Geometry check sheet. Reference: the model listing, model coordinates, mm. Face numbers are marked on the shaded views. A direction names the side the tool comes from. Coordinates: 2 decimals unless noted, no trailing zeros. Order: outer loops, then holes, each group sorted by start corner. A loop starts at its lowest first (then second) coordinate and runs counter-clockwise, first axis right, second up. Notation, with made-up numbers: M 21,-17.5 L 51,-17.5 A6 ccw 51,-12.5 Z; hole C -17.5,46.5 d5. An arc over 180 degrees is marked long. Use CSV: the item, a comma, the result in double quotes. Start each with the question number.
```python
from build123d import *

# Parameters (mm, degrees)
F3_DEPTH = 3.175
F5_DEPTH = 1.27
F6_SIZE2 = 1.27
F6_SIZE  = 0.7332348419


with BuildPart() as f1:
    # F0 (on Top) → F1 (revolve)
    with BuildSketch(Plane.XY):
        Polygon((0, 3.429), (0, 10.2616), (-6.35, 10.2616), (-6.35, 2.38125), (-3.175, 2.38125), (-3.175, 4.191), (-1.905, 4.191), (-1.905, 3.429), align=None)
    revolve(axis=Axis((-3.175, 0, 0), (-1, 0, 0)))

    # F2 (on face) → F3 (cut, through all)
    with BuildSketch(Plane.YZ):
        with BuildLine():
            ThreePointArc((3.429, 0), (2.4246691527, -2.4246691527), (0, -3.429))
            Line((0, -3.429), (9.6717316733, -3.429))
            ThreePointArc((9.6717316733, -3.429), (10.1130578041, -1.7396828477), (10.2616, 0))
            ThreePointArc((10.2616, 0), (10.1130578041, 1.7396828477), (9.6717316733, 3.429))
            Line((9.6717316733, 3.429), (0, 3.429))
            ThreePointArc((0, 3.429), (2.4246691527, 2.4246691527), (3.429, 0))
        make_face()
    extrude(amount=-F3_DEPTH, mode=Mode.SUBTRACT)

    # F4 (on face) → F5 (cut)
    with BuildSketch(Plane.YZ.offset(-3.175)):
        with BuildLine():
            ThreePointArc((0, 4.191), (-4.191, 0), (0, -4.191))
            Line((0, -4.191), (9.3667472241, -4.191))
            ThreePointArc((9.3667472241, -4.191), (9.5268610088, -3.8130504689), (9.6717316733, -3.429))
            ThreePointArc((9.6717316733, -3.429), (10.2616, 0), (9.6717316733, 3.429))
            ThreePointArc((9.6717316733, 3.429), (9.5268610088, 3.8130504689), (9.3667472241, 4.191))
            Line((9.3667472241, 4.191), (0, 4.191))
        make_face()
    extrude(amount=F5_DEPTH, mode=Mode.SUBTRACT)

    # F6
    f6_edges = [f1.edges().sort_by_distance(p)[0] for p in [
        (0, 4.835866, -3.429),
        (0, 4.835866, 3.429),
    ]]
    f6_side = f1.faces().sort_by_distance((0, 4.835866, -3.715101))[0]
    chamfer(f6_edges, length=F6_SIZE, length2=F6_SIZE2, reference=f6_side)


solid = f1.part
```
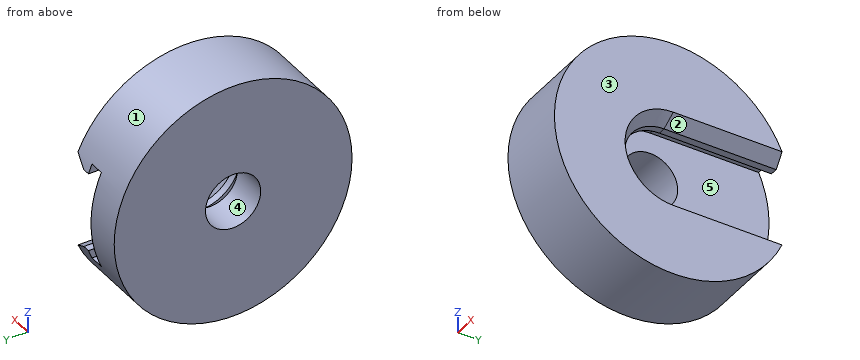
1) Section check B-B on y = 1. Record the boundary of the cut face in (x, z) (3 decimals).
2) Draft check along Z on the marked faces 1, 2 and 3. Enter one of: +Z half, -Z half, draft (parallel to the pull), parting line (faces both ways), or undercut.
3) Section check D-D on y = 3.75. Record the boundary of the cut face in (x, z) (3 decimals), then the cut area to 3 significant figures.
4) Set-up check for the marked faces 4 and 5: record each of +Z, -Z, +X, -X, +Y, -Y from which the full face is reachable in a straight line by a thin tool's end or side.
5) Section check A-A on z = 0. Record the boundary of the cut face in (x, y) (3 decimals), then the cut area to 3 significant figures.
6) Section check C-C on x = -5.5. Record the boundary of the cut face in (y, z), then the cut area to 3 significant figures.
7) Material ranges on line 1 along Z through (x, y) = (-4.8, 0); line 2 along X through (y, z) = (3.75, 1.75) (3 decimals), recorded low to high.
8) Gauge pin test, flat ends, axial feed: P1, Ø4, axis at y = 0, z = 0, coming from the +X side; P2, Ø1, axis at x = -2.5, y = 4, coming from the +Z side; P3, Ø1, axis at x = -3, y = 5.5, coming from the -Z side; P4, Ø3, axis at x = -1.5, y = -7.5, coming from the +Z side. Record the tip position at first contact, or that the pin passes through.
Results are:
1,outline,"M -6.35,-10.213 L 0,-10.213 L 0,-4.162 L -1.27,-3.429 L -1.905,-3.429 L -1.905,-4.191 L -3.175,-4.191 L -3.175,-2.161 L -6.35,-2.161 Z; M -6.35,2.161 L -3.175,2.161 L -3.175,4.191 L -1.905,4.191 L -1.905,3.429 L -1.27,3.429 L 0,4.162 L 0,10.213 L -6.35,10.213 Z"
2,face 1,"parting line"
2,face 2,"undercut"
2,face 3,"draft"
3,outline,"M -6.35,-9.552 L 0,-9.552 L 0,-4.162 L -1.27,-3.429 L -1.905,-3.429 L -1.905,-4.191 L -3.175,-4.191 L -3.175,4.191 L -1.905,4.191 L -1.905,3.429 L -1.27,3.429 L 0,4.162 L 0,9.552 L -6.35,9.552 Z"
3,area,"96.7 mm²"
4,face 4,"+X, -X"
4,face 5,"+Y"
5,outline,"M -6.35,-10.262 L 0,-10.262 L 0,-4.162 L -1.27,-3.429 L -1.905,-3.429 L -1.905,-4.191 L -3.175,-4.191 L -3.175,-2.381 L -6.35,-2.381 Z; M -6.35,2.381 L -3.175,2.381 L -3.175,10.262 L -6.35,10.262 Z"
5,area,"70.3 mm²"
6,outline,"C 0,0 d20.52; hole C 0,0 d4.76"
6,area,"313 mm²"
7,line 1,"z = -10.26 to -2.38, 2.38 to 10.26"
7,line 2,"x = -6.35 to -3.175"
8,P1,"passes through"
8,P2,"stops at z = 9.65"
8,P3,"stops at z = -8.96"
8,P4,"stops at z = 8.32"
